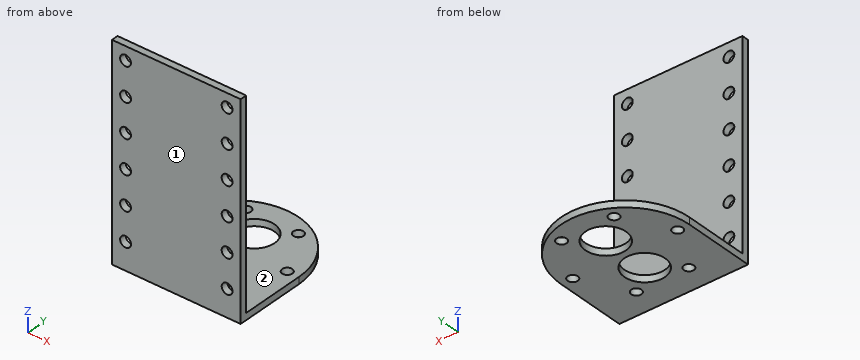
```python
from build123d import *

# Parameters (mm, degrees)
EXTRUDE_1_DEPTH     = 2
SKETCH_2_W          = 38
SKETCH_2_H          = 2
EXTRUDE_2_DEPTH     = 60
SKETCH_3_R          = 1.6
CUT_EXTRUDE_1_DEPTH = 2
SKETCH_4_R          = 6
SKETCH_4_R_2        = 1.5
CUT_EXTRUDE_3_DEPTH = 2


with BuildPart() as part:
    # ｽｹｯﾁ1 → ﾎﾞｽ - 押し出し1 (new body)
    with BuildSketch(Plane.XY):
        with BuildLine():
            Line((-19, 0), (-19, -21))
            Line((-19, -21), (19, -21))
            Line((19, -21), (19, 0))
            ThreePointArc((19, 0), (0, 19), (-19, 0))
        make_face()
    extrude(amount=EXTRUDE_1_DEPTH)

    # ｽｹｯﾁ2 → ﾎﾞｽ - 押し出し2 (add)
    with BuildSketch(Plane.XY.offset(2)):
        with Locations((0, -20)):
            Rectangle(SKETCH_2_W, SKETCH_2_H)
    extrude(amount=EXTRUDE_2_DEPTH)

    # ｽｹｯﾁ3 → ｶｯﾄ - 押し出し1 (cut)
    with BuildSketch(Plane(origin=(0, -19, 0), x_dir=(1, 0, 0), z_dir=(0, 1, 0))):
        with Locations(Location((-15, -8, 0), (0, 0, 270))):  # turned: the seam where the file's is
            Circle(SKETCH_3_R)
        with Locations(Location((-15, -18, 0), (0, 0, 270))):  # turned: the seam where the file's is
            Circle(SKETCH_3_R)
        with Locations(Location((-15, -38, 0), (0, 0, 270))):  # turned: the seam where the file's is
            Circle(SKETCH_3_R)
        with Locations(Location((-15, -28, 0), (0, 0, 270))):  # turned: the seam where the file's is
            Circle(SKETCH_3_R)
        with Locations(Location((-15, -48, 0), (0, 0, 270))):  # turned: the seam where the file's is
            Circle(SKETCH_3_R)
        with Locations(Location((15, -8, 0), (0, 0, 270))):  # turned: the seam where the file's is
            Circle(SKETCH_3_R)
        with Locations(Location((15, -18, 0), (0, 0, 270))):  # turned: the seam where the file's is
            Circle(SKETCH_3_R)
        with Locations(Location((15, -28, 0), (0, 0, 270))):  # turned: the seam where the file's is
            Circle(SKETCH_3_R)
        with Locations(Location((15, -38, 0), (0, 0, 270))):  # turned: the seam where the file's is
            Circle(SKETCH_3_R)
        with Locations(Location((15, -48, 0), (0, 0, 270))):  # turned: the seam where the file's is
            Circle(SKETCH_3_R)
        with Locations(Location((-15, -58, 0), (0, 0, 270))):  # turned: the seam where the file's is
            Circle(SKETCH_3_R)
        with Locations(Location((15, -58, 0), (0, 0, 270))):  # turned: the seam where the file's is
            Circle(SKETCH_3_R)
    extrude(amount=-CUT_EXTRUDE_1_DEPTH, mode=Mode.SUBTRACT)

    # ｽｹｯﾁ4 → ｶｯﾄ - 押し出し3 (cut)
    with BuildSketch(Plane(origin=(0, 0, 0), x_dir=(-1, 0, 0), z_dir=(0, 0, -1))):
        with Locations((0, 7)):
            Circle(SKETCH_4_R)
        with Locations((0, -7)):
            Circle(SKETCH_4_R)
        with Locations((-7.75, 13.423393759)):
            Circle(SKETCH_4_R_2)
        with Locations((-15.5, 0)):
            Circle(SKETCH_4_R_2)
        with Locations((15.5, 0)):
            Circle(SKETCH_4_R_2)
        with Locations((7.75, 13.423393759)):
            Circle(SKETCH_4_R_2)
        with Locations((7.75, -13.423393759)):
            Circle(SKETCH_4_R_2)
        with Locations((-7.75, -13.423393759)):
            Circle(SKETCH_4_R_2)
    extrude(amount=-CUT_EXTRUDE_3_DEPTH, mode=Mode.SUBTRACT)


solid = part.part
```
Input: part model. Units: mm. Frame: model coordinates. Face numbers are marked on the shaded views. A direction names the side the tool comes from. Coordinates: 2 decimals unless noted, no trailing zeros. Loops run counter-clockwise (first coordinate to the right, second up) from the corner with the lowest first, then second, coordinate; pieces in that order, holes last.
Q1. Section A-A, the plane z = 58. Return the cut outline in (x, y).
Results are:
outline: (-19, -21) - (-16.6, -21) - (-16.6, -19) - (-19, -19) - close; (-13.4, -21) - (13.4, -21) - (13.4, -19) - (-13.4, -19) - close; (16.6, -21) - (19, -21) - (19, -19) - (16.6, -19) - close
Q2. Section B-B, the plane x = 1.5. Return the cut outline in (y, z).
Results are:
outline: (-21, 0) - (-12.81, 0) - (-12.81, 2) - (-19, 2) - (-19, 62) - (-21, 62) - close; (-1.19, 0) - (1.19, 0) - (1.19, 2) - (-1.19, 2) - close; (12.81, 0) - (18.94, 0) - (18.94, 2) - (12.81, 2) - close
Q3. Section C-C, the plane y = 7. Return the cut outline in (x, z), and give its area (3 significant figures).
Results are:
outline: (-17.66, 0) - (-6, 0) - (-6, 2) - (-17.66, 2) - close; (6, 0) - (17.66, 0) - (17.66, 2) - (6, 2) - close
area: 46.7 mm2
Q4. Set-up query: the marked faces 1 and 2. Return all of +Z, -Z, +X, -X, +Y, -Y with unobstructed straight access to the full face (end or side cutting, diameter ignored); none if empty.
Results are:
face 1: +Z, -Z, +X, -X, -Y
face 2: +Z, +X, -X, +Y
Q5. Line query: line 1 along X through (y, z) = (-20.5, 18); line 2 along Y through (x, z) = (0, 1); line 3 along Z through (x, y) = (6, -18). Output: solid intervals per line, ascending.
Results are:
line 1: x = -19 to -16.6, -13.4 to 13.4, 16.6 to 19
line 2: y = -21 to -13, -1 to 1, 13 to 19
line 3: z = 0 to 2
Q6. Contact query for flat-ended pins moving along their axis: pin 1 (5 mm diameter, centred on x = -15, z = 48, fed in from +Y); pin 2 (2.5 mm diameter, centred on x = -15, z = 28, fed in from +Y); pin 3 (4 mm diameter, centred on x = -15.5, y = 0, fed in from +Z); pin 4 (5 mm diameter, centred on x = 7.75, y = 13.42, fed in from -Z). Output: stop coordinate, or through.
Results are:
pin 1: stops at y = -19
pin 2: passes through
pin 3: stops at z = 2
pin 4: stops at z = 0
Q7. Section D-D, the plane x = -15. Give the number of separate pieces and of enclosed holes in the cut face, and give its area (3 significant figures).
Results are:
separate pieces: 8
enclosed holes: 0
area: 141 mm2
